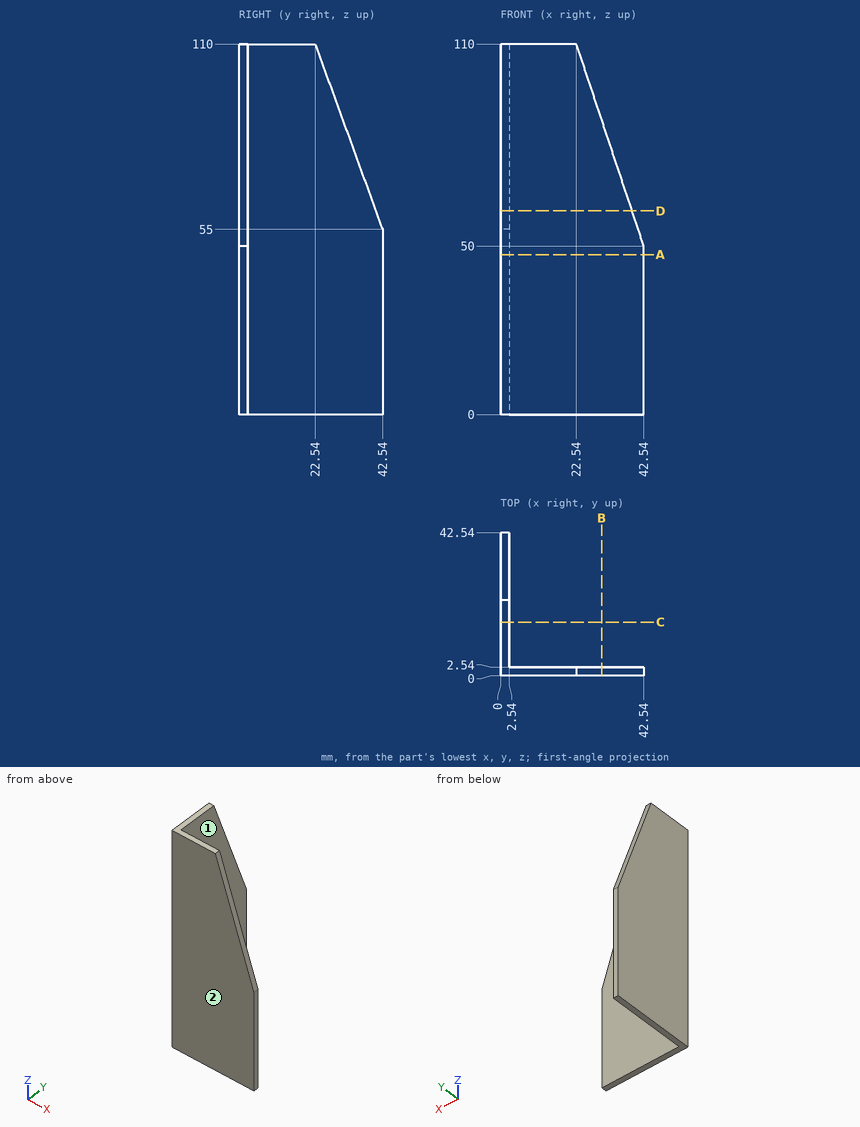
Print and shaded views of the part. All mm, measured from the part's lowest x, y and z. A direction names the side the tool comes from. Coordinates: 2 decimals unless noted, no trailing zeros. Order: outer loops, then holes, each group sorted by start corner. A loop starts at its lowest first (then second) coordinate and runs counter-clockwise, first axis right, second up. Notation, with made-up numbers: M -39,40 L 12,40 A26 cw 12,67 Z; hole C -2,48 d3. An arc over 180 degrees is marked long. Write each question's results on one line, items separated by ' | '. Start each with the question number.
Q1. Which spindle directions (+Z, -Z, +X, -X, +Y, -Y) get a long thin tool onto all of the face, cutting with end or side? Do the marked faces 1 and 2. Say none if no direction does.
Q2. Cut at A-A (z = 47.5). List the corners of the cut face in (x, y), then the cut area to 3 significant figures.
Q3. Cut at D-D (z = 60.5). List the corners of the cut face in (x, y), then the cut area to 3 significant figures.
Q4. Flat gauge pins, fed straight in: P1, Ø6, axis at x = 6, z = 72, coming from the +Y side; P2, Ø10, axis at y = 16.5, z = 56, coming from the +X side; P3, Ø3, axis at y = 32, z = 91, coming from the +X side. Where does each tip first touch, or does it go through?
Q5. Cut at B-B (x = 30). List the corners of the cut face in (y, z).
Q6. Cut at C-C (y = 16). List the corners of the cut face in (x, z).
Q7. Drill centre lines: probe 1 along Y at (x, z) = (28, 24); probe 2 along X at (y, z) = (2.5, 75). Where is each one in solid material? Low to high. Write a range as from..to.
Found:
1) face 1: +Z, -Z, +X, +Y | face 2: +Z, -Z, +X, -X, -Y
2) outline: M 0,0 L 42.54,0 L 42.54,2.54 L 2.54,2.54 L 2.54,42.54 L 0,42.54 Z | area: 210 mm²
3) outline: M 0,0 L 39.04,0 L 39.04,2.54 L 2.54,2.54 L 2.54,40.54 L 0,40.54 Z | area: 196 mm²
4) P1: y = 2.54 | P2: x = 2.54 | P3: through
5) outline: M 0,0 L 2.54,0 L 2.54,87.62 L 0,87.62 Z
6) outline: M 0,0 L 2.54,0 L 2.54,110 L 0,110 Z
7) probe 1: 0..2.54 | probe 2: 0..34.21
